```python
from build123d import *

# Parameters (mm, degrees)
F0_R      = 12.5
F1_DEPTH  = 70
F2_W      = 75
F2_H      = 15
F3_DEPTH  = 175
F4_W      = 25
F4_H      = 145
F5_DEPTH  = 500
F6_W      = 75
F6_H      = 20
F7_DEPTH  = 50
F8_R      = 5
F9_DEPTH  = 20
F10_R     = 5
F11_DEPTH = 20


with BuildPart() as f1:
    # F0 (on Right) → F1 (new body, symmetric)
    with BuildSketch(Plane.YZ):
        Circle(F0_R)
    extrude(amount=F1_DEPTH, both=True)

    # F2 (on Top) → F3 (join)
    with BuildSketch(Plane.XY):
        Rectangle(F2_W, F2_H)
    extrude(amount=F3_DEPTH)

    # F4 (on face) → F5 (cut)
    with BuildSketch(Plane.XZ.offset(7.5)):
        with Locations((-12.5, 82.5)):
            Rectangle(F4_W, F4_H)
        with Locations((12.5, 82.5)):
            Rectangle(F4_W, F4_H)
    extrude(amount=-F5_DEPTH, mode=Mode.SUBTRACT)

    # F6 (on face) → F7 (join)
    with BuildSketch(Plane.XZ.offset(7.5)):
        with Locations((0, 165)):
            Rectangle(F6_W, F6_H)
    extrude(amount=-F7_DEPTH)

    # F8 (on face) → F9 (cut)
    with BuildSketch(Plane(origin=(-37.5, 0, 0), x_dir=(0, -1, 0), z_dir=(-1, 0, 0))):
        with Locations((-32.5, 165)):
            Circle(F8_R)
    extrude(amount=-F9_DEPTH, mode=Mode.SUBTRACT)

    # F10 (on face) → F11 (cut)
    with BuildSketch(Plane.YZ.offset(37.5)):
        with Locations((32.5, 165)):
            Circle(F10_R)
    extrude(amount=-F11_DEPTH, mode=Mode.SUBTRACT)


solid = f1.part
```
CAD build for the part. Positions are in the model's coordinates, mm. A direction names the side the tool comes from. Round coordinates to 2 decimals unless told otherwise and drop trailing zeros. Order: outer loops, then holes, each group sorted by start corner. A loop starts at its lowest first (then second) coordinate and runs counter-clockwise, first axis right, second up.
Item 1: Saw through at A-A on x = -34. Write the cut outline in (y, z), then the cut area to 3 significant figures.
Item 2: Pin check, flat tips, straight feed: pin 1 (15 mm diameter, centred on x = 0.5, y = 17.5, fed in from -Z); pin 2 (16.5 mm diameter, centred on y = 1.5, z = 66, fed in from -X); pin 3 (7.5 mm diameter, centred on y = 3.5, z = 74, fed in from +X). Stop position of each tip, or through.
Item 3: Saw through at C-C on z = 57.5. Write the cut outline in (x, y), then the cut area to 3 significant figures.
Item 4: Mould opens along Z. For faces 1 (the face through (0, 0, 10)), 2 (the face through (31, 7.5, 81)), 3 (the face through (-1, 18, 175)), 4 (the face through (-70, 0, 0)) say: pulls with the +Z half, pulls with the -Z half, needs draft (parallel to the pull), parting line crosses it, or undercut.
Item 5: Tool access for faces 5 (the face through (-31, 7.5, 81)), 6 (the face through (-26, -7.5, 110)), 7 (the face through (27.64, 31.849, 169.957)), 8 (the face through (-1, 17, 155)): list every direction of +Z, -Z, +X, -X, +Y, -Y with a clear straight run to the whole face (end or side of a thin tool).
Item 6: Saw through at D-D on y = 0. Write the cut outline in (x, z).
Item 7: Probe line 1 along Z through (x, y) = (25, 32.5); line 2 along Z through (x, y) = (10, 0); line 3 along X through (y, z) = (1, 124). List the from-to ranges inside material, lowest first.
Item 8: Saw through at B-B on y = 10. Write the cut outline in (x, z).
Reported:
1. outline: (-7.5, 10) arc R12.5 ccw (long way) to (7.5, 10) - (7.5, 155) - (42.5, 155) - (42.5, 175) - (-7.5, 175) - close; hole circle Ø10 at (32.5, 165)
1. area: 3,560 mm2
2. pin 1: stops at z = -7.5
2. pin 2: stops at x = -37.5
2. pin 3: stops at x = 37.5
3. outline: (-37.5, -7.5) - (-25, -7.5) - (-25, 7.5) - (-37.5, 7.5) - close; (25, -7.5) - (37.5, -7.5) - (37.5, 7.5) - (25, 7.5) - close
3. area: 375 mm2
4. face 1: undercut
4. face 2: undercut
4. face 3: pulls with the +Z half
4. face 4: needs draft
5. face 5: +X, -X, +Y
5. face 6: +Z, +X, -X, -Y
5. face 7: +X
5. face 8: +Y
6. outline: (-70, -12.5) - (70, -12.5) - (70, 12.5) - (37.5, 12.5) - (37.5, 175) - (-37.5, 175) - (-37.5, 12.5) - (-70, 12.5) - close; hole (-25, 10) - (25, 10) - (25, 155) - (-25, 155) - close
7. line 1: z = 155 to 160, 170 to 175
7. line 2: z = -12.5 to 10, 155 to 175
7. line 3: x = -37.5 to -25, 25 to 37.5
8. outline: (-70, -7.5) - (70, -7.5) - (70, 7.5) - (-70, 7.5) - close; (-37.5, 155) - (37.5, 155) - (37.5, 175) - (-37.5, 175) - close
